For this review, take the finished solid that the model builds, in its own axes (mm). A direction names the side the tool comes from. Give positions to 0.01 mm unless a question says otherwise; leave off trailing zeros. Order: outer loops, then holes, each group sorted by start corner. A loop starts at its lowest first (then second) coordinate and runs counter-clockwise, first axis right, second up. Notation, with made-up numbers: M -5.5,2.5 L 20.5,2.5 A31 ccw 20.5,31.5 Z; hole C -35,29.5 d8. An arc over 180 degrees is marked long. Answer as CSV lines item,"result". Start each with the question number.
1. We need section A-A, the plane y = 11. Give the boundary of the cut face in (x, z).
2. Clearance check with flat-ended pins moving along their axes: P1, Ø3, axis at x = 13, z = 7, coming from the +Y side; P2, Ø1.5, axis at y = 25.5, z = 8.5, coming from the +X side; P3, Ø1.5, axis at x = 4.5, z = 3, coming from the +Y side; P4, Ø4, axis at x = -6.6, y = 12.21, coming from the -Z side. State where each tip first meets the part, or that it passes through.
3. We need section B-B, the plane x = -7. Give the boundary of the cut face in (y, z), and give its area (3 significant figures).
4. We need section D-D, the plane y = 3.5. Give the boundary of the cut face in (x, z), and give its area (3 significant figures).
5. For line 1 along X through (y, z) = (-2, 3.5); line 2 along Z through (x, y) = (0.5, 0); line 3 along Y through (x, z) = (-7.5, 3.5), list the stretches that pass through material, from the lowest coordinate up.
6. Mouldability with a two-part tool opening along Y and no side actions: class faces 4 (the flat face through (7, -1, 9.092)), 5 (the flat face through (11.195, -4, 6)), 6 (the cylindrical face through (25.06, 30.4, 6.18)) as pulls with the +Y half, pulls with the -Y half, needs draft (parallel to the pull), parting line crosses it, or undercut.
7. We need section C-C, the plane z = 6.5. State how many separate pieces and enclosed holes the cut face has, and give its area (3 significant figures).
8. Machinability: for faces 1 (the flat face through (-0.976, 0, 6)), 2 (the flat face through (7, 2.979, 6)), 3 (the flat face through (-5.15, 7.644, 6.177)), which of the approach directions +Z, -Z, +X, -X, +Y, -Y give a long, thin tool a straight path to every point of the face, cutting with its end or side? Answer none if there is none.
from build123d import *

# Parameters (mm, degrees)
SKETCH1_R               = 2.6162
BOSS_EXTRUDE1_DEPTH     = 8.255
BOSS_EXTRUDE2_START     = -8.255
BOSS_EXTRUDE2_DEPTH     = 8.255
CUT_EXTRUDE1_DEPTH      = 48.016961983
CUT_EXTRUDE1_DEPTH_BACK = 1.397
SKETCH3_W               = 8.255
SKETCH3_H               = 6.985
BOSS_EXTRUDE3_DEPTH     = 1.27


with BuildPart() as part:
    # Sketch1 → Boss-Extrude1 (new body)
    with BuildSketch(Plane.XY.offset(2.107322193)):
        with BuildLine():
            Line((-0.976083412, 8.428441548), (0.293916588, 8.428441851))
            Line((0.293916588, 8.428441851), (0.293916229, 9.932994282))
            ThreePointArc((0.293916229, 9.932994282), (-0.000418872, 12.651350758), (-0.869779891, 15.243706156))
            Line((-0.869779891, 15.243706156), (-0.976085093, 15.474629701))
            ThreePointArc((-0.976085093, 15.474629701), (6.540220685, 27.79826422), (15.111028831, 16.183270977))
            Line((15.111028831, 16.183270977), (14.582439814, 14.704895001))
            ThreePointArc((14.582439814, 14.704895001), (14.027755034, 12.598915738), (13.841030203, 10.42913287))
            Line((13.841030203, 10.42913287), (13.84103068, 8.428445081))
            Line((13.84103068, 8.428445081), (15.11103068, 8.428445384))
            Line((15.11103068, 8.428445384), (15.111029589, 13.002746336))
            ThreePointArc((15.111029589, 13.002746336), (15.312546971, 14.115862595), (15.891518981, 15.087679694))
            Line((15.891518981, 15.087679694), (24.488045189, 24.960647863))
            ThreePointArc((24.488045189, 24.960647863), (25.020724695, 30.469297747), (19.983753108, 32.762306303))
            Line((19.983753108, 32.762306303), (5.247640051, 29.885468019))
            ThreePointArc((5.247640051, 29.885468019), (2.188775836, 28.740388475), (-0.332323255, 26.663872928))
            Line((-0.332323255, 26.663872928), (-10.19178942, 15.340439107))
            ThreePointArc((-10.19178942, 15.340439107), (-10.724468925, 9.831789223), (-5.687497339, 7.538780667))
            Line((-5.687497339, 7.538780667), (-4.598119195, 7.751453082))
            ThreePointArc((-4.598119195, 7.751453082), (-2.818463394, 8.257741333), (-0.976083412, 8.428441548))
        make_face()
        with Locations((-6.600023508, 12.213040207)):
            Circle(SKETCH1_R, mode=Mode.SUBTRACT)
        with Locations((20.896279277, 28.088046763)):
            Circle(SKETCH1_R, mode=Mode.SUBTRACT)
    extrude(amount=BOSS_EXTRUDE1_DEPTH)

    # Sketch2 → Boss-Extrude2 (add)
    with BuildSketch(Plane.XY.offset(10.362322193).offset(BOSS_EXTRUDE2_START)):
        with BuildLine():
            Line((0.293916229, 9.932991253), (0.293916588, 8.428441851))
            Line((0.293916588, 8.428441851), (-0.976083412, 8.428441548))
            ThreePointArc((-0.976083412, 8.428441548), (-2.818463394, 8.257741333), (-4.598119195, 7.751453082))
            ThreePointArc((-4.598119195, 7.751453082), (-2.387631267, 7.376407845), (-0.976082746, 5.634441548))
            Line((-0.976082746, 5.634441548), (-0.976080172, -5.160558452))
            Line((-0.976080172, -5.160558452), (15.11103392, -5.160554616))
            Line((15.11103392, -5.160554616), (15.11103068, 8.428445384))
            Line((15.11103068, 8.428445384), (13.84103068, 8.428445081))
            Line((13.84103068, 8.428445081), (13.841030203, 10.42913287))
            ThreePointArc((13.841030203, 10.42913287), (14.027755034, 12.598915738), (14.582439814, 14.704895001))
            Line((14.582439814, 14.704895001), (15.111028831, 16.183270977))
            ThreePointArc((15.111028831, 16.183270977), (6.540220685, 27.79826422), (-0.976085093, 15.474629701))
            Line((-0.976085093, 15.474629701), (-0.869779891, 15.243706156))
            ThreePointArc((-0.869779891, 15.243706156), (-0.000418548, 12.651349279), (0.293916229, 9.932991253))
        make_face()
        Polygon((0.293917905, 2.903941851), (0.293916588, 2.979402319), (13.841031997, 2.979402319), (13.841031997, 2.903945081), (13.841033587, -3.763554919), (0.293919495, -3.763558149), align=None, mode=Mode.SUBTRACT)
    extrude(amount=BOSS_EXTRUDE2_DEPTH)

    # Sketch3 → Cut-Extrude1 (cut, two sides: drawn at the far end of the back side and taken through both)
    with BuildSketch(Plane(origin=(1.231e-06, -5.160558219, 0), x_dir=(0.9999999999999716, 2.3845959458266363e-07, 0), z_dir=(2.3845959458266363e-07, -0.9999999999999716, 0)).offset(-CUT_EXTRUDE1_DEPTH_BACK)):
        with Locations((7.067475644, 5.599822193)):
            Rectangle(SKETCH3_W, SKETCH3_H)
    extrude(amount=CUT_EXTRUDE1_DEPTH + CUT_EXTRUDE1_DEPTH_BACK, mode=Mode.SUBTRACT)

    # Sketch4 → Boss-Extrude3 (add)
    with BuildSketch(Plane.XY.offset(10.362322193)):
        Polygon((13.841031997, 2.903945081), (13.841031997, 2.979402319), (0.293916588, 2.979402319), (0.293917905, 2.903941851), (0.293919495, -3.763558149), (13.841033587, -3.763554919), align=None)
    extrude(amount=-BOSS_EXTRUDE3_DEPTH)


solid = part.part
Result set:
1,outline,"M -11.21,2.11 L -8.92,2.11 L -8.92,10.36 L -11.21,10.36 Z; M -4.28,2.11 L 15.11,2.11 L 15.11,10.36 L -4.28,10.36 Z"
2,P1,"y = 31.69"
2,P2,"x = 25.29"
2,P3,"y = 29.89"
2,P4,"through"
3,outline,"M 7.47,2.11 L 9.63,2.11 L 9.63,10.36 L 7.47,10.36 Z; M 14.8,2.11 L 19.01,2.11 L 19.01,10.36 L 14.8,10.36 Z"
3,area,"52.6 mm2"
4,outline,"M -0.98,2.11 L 15.11,2.11 L 15.11,10.36 L -0.98,10.36 Z"
4,area,"133 mm2"
5,line 1,"-0.98 to 0.29, 13.84 to 15.11"
5,line 2,"9.09 to 10.36"
5,line 3,"7.54 to 9.76, 14.67 to 18.43"
6,face 4,"undercut"
6,face 5,"needs draft"
6,face 6,"parting line crosses it"
7,separate pieces,"1"
7,enclosed holes,"2"
7,area,"668 mm2"
8,face 1,"+Z, -Z, -X, -Y"
8,face 2,"-Z"
8,face 3,"+Z, -Z, -Y"
